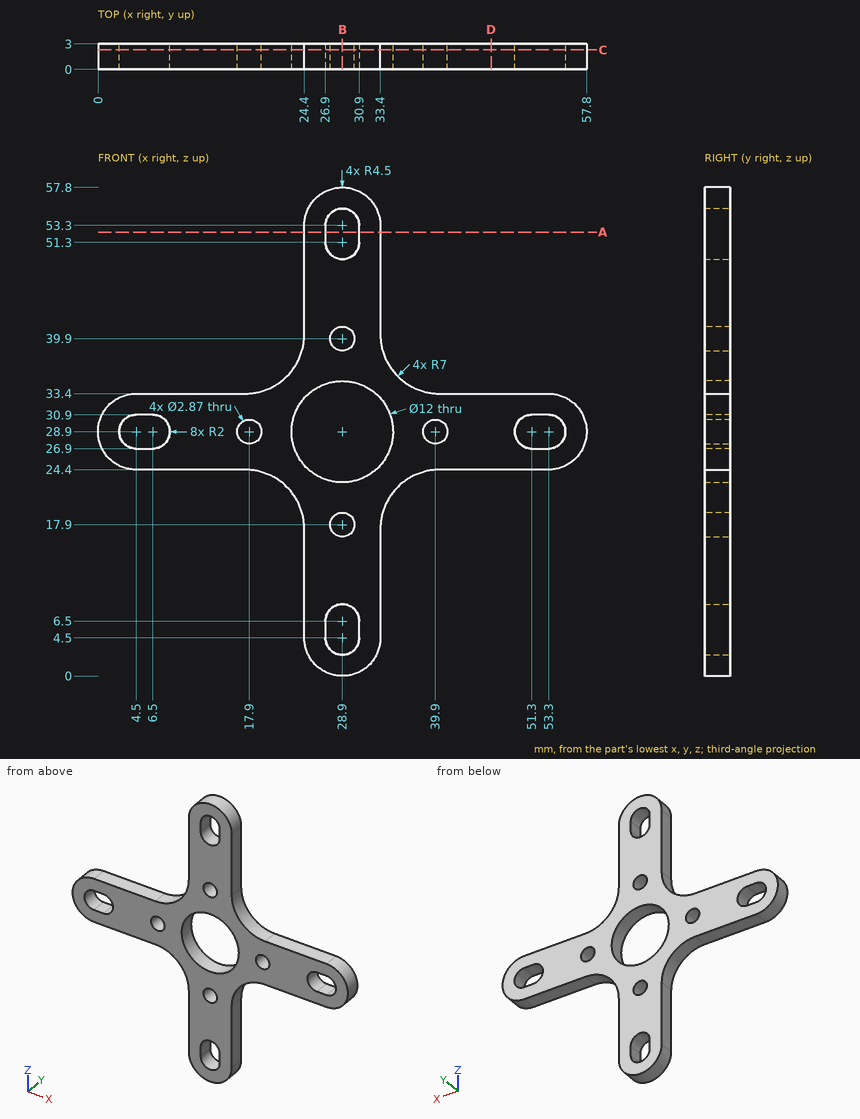
Source: three-view drawing plus pictorial views. Frame: mm from the lowest corner of the part. Round coordinates to 2 decimals unless told otherwise and drop trailing zeros. Write each loop counter-clockwise with the first axis right and the second up, starting at its lowest first coordinate (ties: lowest second). Pieces come first, ordered by that corner, then holes. Notation, with made-up numbers: M 83.5,74.5 L 122.5,74.5 A19 ccw 122.5,85.5 Z; hole C 32.5,-24 d11. An arc over 180 degrees is marked long. Use CSV: the item, a comma, the result in double quotes. Start each with the question number.
Q1. Line query: line 1 (X direction, y = 0.8, z = 28.9) (1 decimal); line 2 (Z direction, x = 28.5, y = 0.3); line 3 (X direction, y = 1.6, z = 4). Output: solid intervals per line, ascending. Write a range as from..to.
Q2. Cut plane B-B on x = 28.9. Output: boundary loops of the cut face in (y, z) (1 decimal).
Q3. Cut plane C-C on y = 2.3. Count the separate pieces of the cut face and the enclosed holes in it.
Q4. First-contact query: P1, Ø0.9, axis at y = 1, z = 46, coming from the +X side; P2, Ø1, axis at x = 32, y = 1.5, coming from the +Z side; P3, Ø0.9, axis at x = 49.5, y = 1.5, coming from the -Z side. Flat tips, straight axial feed; report the tip coordinate or a pass-through.
Q5. Cut plane D-D on x = 46.5. Output: boundary loops of the cut face in (y, z), plus the area to 3 significant figures.
Q6. Cut plane A-A on z = 52.5. Output: boundary loops of the cut face in (x, y).
Results found:
1,line 1,"0..2.5, 8.5..16.5, 19.3..22.9, 34.9..38.5, 41.3..49.3, 55.3..57.8"
1,line 2,"0.02..2.54, 8.46..16.52, 19.28..22.91, 34.89..38.52, 41.28..49.34, 55.26..57.78"
1,line 3,"24.43..26.96, 30.84..33.37"
2,outline,"M 0,0 L 3,0 L 3,2.5 L 0,2.5 Z; M 0,8.5 L 3,8.5 L 3,16.5 L 0,16.5 Z; M 0,19.3 L 3,19.3 L 3,22.9 L 0,22.9 Z; M 0,34.9 L 3,34.9 L 3,38.5 L 0,38.5 Z; M 0,41.3 L 3,41.3 L 3,49.3 L 0,49.3 Z; M 0,55.3 L 3,55.3 L 3,57.8 L 0,57.8 Z"
3,separate pieces,"1"
3,enclosed holes,"9"
4,P1,"x = 33.4"
4,P2,"z = 56.97"
4,P3,"z = 24.4"
5,outline,"M 0,24.4 L 3,24.4 L 3,33.4 L 0,33.4 Z"
5,area,"27.0 mm^2"
6,outline,"M 24.4,0 L 26.9,0 L 26.9,3 L 24.4,3 Z; M 30.9,0 L 33.4,0 L 33.4,3 L 30.9,3 Z"
